```python
from build123d import *

# Parameters (mm, degrees)
F1_DEPTH       = 190
F2_SIZE        = 2
F4_D           = 6
F5_D           = 11
F5_CSINK_D     = 20.5
F5_CSINK_ANGLE = 90


with BuildPart() as f1:
    # F0 (on Right) → F1 (new body, symmetric)
    with BuildSketch(Plane.YZ):
        Polygon((19, 13), (-19, 13), (-19, 3.5), (-37.5, 3.5), (-37.5, -13), (37.5, -13), (37.5, 3.5), (19, 3.5), align=None)
    extrude(amount=F1_DEPTH, both=True)

    # F2
    f2_edges = [f1.edges().sort_by_distance(p)[0] for p in [
        (0, -37.5, -13),
        (-190, 0, -13),
        (0, 37.5, -13),
        (190, 0, -13),
        (-190, 0, 13),
        (0, -19, 13),
        (190, 0, 13),
        (0, 19, 13),
        (0, -37.5, 3.5),
        (0, 37.5, 3.5),
        (190, 28.25, 3.5),
        (190, -28.25, 3.5),
        (-190, -28.25, 3.5),
        (-190, 28.25, 3.5),
    ]]
    chamfer(f2_edges, length=F2_SIZE)

    # F4 (through all)
    with Locations(Plane.XY.offset(13)):
        with Locations((0, 0)):
            Hole(F4_D / 2)

    # F5 (through all)
    with Locations(Plane.XY.offset(13)):
        with Locations((-136, 0), (-60, 0), (60, 0), (136, 0)):
            CounterSinkHole(F5_D / 2, F5_CSINK_D / 2, counter_sink_angle=F5_CSINK_ANGLE)


solid = f1.part
```
Can you work these out from the model? Positions are in its coordinate system, mm. A direction names the side the tool comes from. Coordinates: 2 decimals unless noted, no trailing zeros. Loops run counter-clockwise (first coordinate to the right, second up) from the corner with the lowest first, then second, coordinate; pieces in that order, holes last.
Item 1: Suppose I cut it at B-B (x = -136). Please give me the cut outline in (y, z), then the cut area to 3 significant figures.
Answers below:
outline: (-37.5, -11) - (-35.5, -13) - (-5.5, -13) - (-5.5, 8.25) - (-10.25, 13) - (-17, 13) - (-19, 11) - (-19, 3.5) - (-35.5, 3.5) - (-37.5, 1.5) - close; (5.5, -13) - (35.5, -13) - (37.5, -11) - (37.5, 1.5) - (35.5, 3.5) - (19, 3.5) - (19, 11) - (17, 13) - (10.25, 13) - (5.5, 8.25) - close
area: 1,280 mm2
Item 2: Suppose I cut it at C-C (y = 30). Please give me the cut outline in (x, z), then the cut area to 3 significant figures.
Answers below:
outline: (-190, -11) - (-188, -13) - (188, -13) - (190, -11) - (190, 1.5) - (188, 3.5) - (-188, 3.5) - (-190, 1.5) - close
area: 6,260 mm2
Item 3: I'm going to push flat-ended pins straight in: pin 1 (14.5 mm diameter, centred on x = -136, y = 0, fed in from +Z); pin 2 (5.5 mm diameter, centred on x = 0, y = 0, fed in from +Z); pin 3 (17.5 mm diameter, centred on x = -60, y = 0, fed in from +Z); pin 4 (17.5 mm diameter, centred on x = 60, y = 0, fed in from -Z). Where does each tip first touch, or does it pass through?
Answers below:
pin 1: stops at z = 10
pin 2: passes through
pin 3: stops at z = 11.5
pin 4: stops at z = -13
Item 4: Suppose I cut it at A-A (x = -22). Please give me the cut outline in (y, z), then the cut area to 3 significant figures.
Answers below:
outline: (-37.5, -11) - (-35.5, -13) - (35.5, -13) - (37.5, -11) - (37.5, 1.5) - (35.5, 3.5) - (19, 3.5) - (19, 11) - (17, 13) - (-17, 13) - (-19, 11) - (-19, 3.5) - (-35.5, 3.5) - (-37.5, 1.5) - close
area: 1,590 mm2
Item 5: If we mould it in two halves opening along X, with no side actions, what happens to faces 1 (the face through (-130.505, 0.242, -2.524)), 2 (the face through (3, 37.5, -5)), 3 (the face through (-190, -1, -2)), 4 (the face through (141.725, 0.252, 8.481))? For each: released by +X, released by -X, zero draft, split by the parting line, or undercut.
Answers below:
face 1: undercut
face 2: zero draft
face 3: released by -X
face 4: undercut
Item 6: Please list where these lines run through material, in increasing order: L1, parallel to Y at x = 0, z = 7.25; L2, parallel to Y at x = 0, z = -4.25; L3, parallel to X at y = -4.5, z = 7.5.
Answers below:
L1: y = -19 to -3, 3 to 19
L2: y = -37.5 to -3, 3 to 37.5
L3: x = -190 to -139.16, -132.84 to -63.16, -56.84 to 56.84, 63.16 to 132.84, 139.16 to 190
Item 7: Which directions (+Z, -Z, +X, -X, +Y, -Y) give clear straight access to the entire face, cutting with the end or side of a thin tool? Please do faces 5 (the face through (3, -27, 3.5)), 6 (the face through (-54.505, 0.242, -2.524)), 7 (the face through (3, 27, 3.5)).
Answers below:
face 5: +Z, +X, -X, -Y
face 6: +Z, -Z
face 7: +Z, +X, -X, +Y
